Check sheet for the modelled part. Datum: model origin and axes. Units: mm. Give positions to 0.01 mm unless a question says otherwise; leave off trailing zeros. Loops run counter-clockwise (first coordinate to the right, second up) from the corner with the lowest first, then second, coordinate; pieces in that order, holes last. Notation, with made-up numbers: (-18, 62.25) - (4, 62.25) arc R13 cw to (4, 81.25) - close; hole circle Ø7 at (60, 59). An arc over 180 degrees is marked (long way). Use CSV: the item, a comma, the result in double quotes.
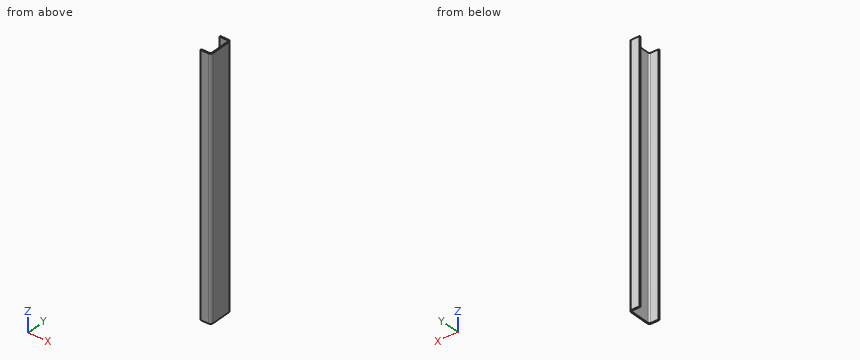
from build123d import *

# Parameters (mm, degrees)
BASE_EXTRUDE_THIN_DEPTH = 2133.6
INSIDE_BEND_RADIUS_R    = 12.7
OUTSIDE_BEND_RADIUS_R   = 22.225


with BuildPart() as part:
    # Sketch1 → Base-Extrude-Thin (new body)
    with BuildSketch(Plane.XY):
        Polygon((-88.9, 0), (0, 0), (0, 209.55), (-88.9, 209.55), (-88.9, 200.025), (-9.525, 200.025), (-9.525, 9.525), (-88.9, 9.525), align=None)
    extrude(amount=-BASE_EXTRUDE_THIN_DEPTH)

    # Inside Bend Radius
    inside_bend_radius_edges = [part.edges().sort_by_distance(p)[0] for p in [
        (-9.525, 200.025, -1066.8),
        (-9.525, 9.525, -1066.8),
    ]]
    fillet(inside_bend_radius_edges, radius=INSIDE_BEND_RADIUS_R)

    # Outside Bend Radius
    outside_bend_radius_edges = [part.edges().sort_by_distance(p)[0] for p in [
        (0, 0, -1066.8),
        (0, 209.55, -1066.8),
    ]]
    fillet(outside_bend_radius_edges, radius=OUTSIDE_BEND_RADIUS_R)


solid = part.part
1. Sectioned sample at C-C, the plane y = 89. Record the boundary of the cut face in (x, z) (3 decimals).
Completed:
outline,"(-9.525, -2133.6) - (0, -2133.6) - (0, 0) - (-9.525, 0) - close"
2. Sectioned sample at A-A, the plane x = -50. Record the boundary of the cut face in (y, z) (3 decimals), and give its area (3 significant figures).
Completed:
outline,"(0, -2133.6) - (9.525, -2133.6) - (9.525, 0) - (0, 0) - close; (200.025, -2133.6) - (209.55, -2133.6) - (209.55, 0) - (200.025, 0) - close"
area,"40,600 mm²"
3. Sectioned sample at B-B, the plane z = -1034.5. Record the boundary of the cut face in (x, y) (3 decimals), and give its area (3 significant figures).
Completed:
outline,"(-88.9, 0) - (-22.225, 0) arc R22.225 ccw to (0, 22.225) - (0, 187.325) arc R22.225 ccw to (-22.225, 209.55) - (-88.9, 209.55) - (-88.9, 200.025) - (-22.225, 200.025) arc R12.7 cw to (-9.525, 187.325) - (-9.525, 22.225) arc R12.7 cw to (-22.225, 9.525) - (-88.9, 9.525) - close"
area,"3,370 mm²"
4. Scan lines: line 1 along Y through (x, z) = (-63, -1105) (3 decimals); line 2 along X through (y, z) = (124, -1634) (3 decimals); line 3 along Y through (x, z) = (-16, -900). Record each from-to range of solid material in increasing order.
Completed:
line 1,"y = 0 to 9.525, 200.025 to 209.55"
line 2,"x = -9.525 to 0"
line 3,"y = 0.89 to 11.16, 198.39 to 208.66"
5. Go/stop test with a flat-tipped pin: pin 1 Ø10 at (y, z) = (65.5, -468.5) entering from -X (3 decimals). Record where the tip stops, or that it passes through.
Completed:
pin 1,"stops at x = -9.525"
